The listing builds one solid part. Answer for the finished solid, in the listing's coordinates (mm). A direction names the side the tool comes from. Round coordinates to 2 decimals unless told otherwise and drop trailing zeros. Write each loop counter-clockwise with the first axis right and the second up, starting at its lowest first coordinate (ties: lowest second). Pieces come first, ordered by that corner, then holes. Notation, with made-up numbers: M 50,-19.75 L 96,-19.75 A29 cw 96,16.25 Z; hole C 19,2.5 d4. An arc over 180 degrees is marked long. One line per item, written item: value. Start each with the question number.
(1) Consider probe 1 along Y at (x, z) = (6.25, -1) (3 decimals); probe 2 along Z at (x, y) = (6.25, 2.4) (1 decimal); probe 3 along Z at (x, y) = (11.25, -18.5). Determine where each line is inside the solid, lowest interval first.
(2) Section D-D (x = 10.75) is taken. Determine the outline of the cut face in (y, z) (3 decimals).
(3) For faces 5 (the flat face through (6, -10, -2)), 6 (the flat face through (9, -19.094, -1)), 7 (the flat face through (6, 5, -7)), determine the directions among +Z, -Z, +X, -X, +Y, -Y from which every point of the face is accessible in a straight line to the end or side of a thin tool.
(4) Given P1, Ø3, axis at x = 2, y = -9.5, coming from the -Z side; P2, Ø6, axis at x = 4, z = -9, coming from the -Y side; P3, Ø1, axis at x = 7.5, z = -0.5, coming from the -Y side, each flat-ended and moving along its own axis, determine where each tip first touches the part or whether it passes through.
(5) Section C-C (z = -8) is taken. Determine the outline of the cut face in (x, y).
(6) For a pull along X with two mould halves and no side action, classify faces 1 (the flat face through (12.5, 1, -7)), 2 (the cylindrical face through (6.429, -14.387, -1.014)), 3 (the flat face through (0, 1, -6)), 4 (the flat face through (6, 2, -17.135)) as released by +X, released by -X, zero draft, split by the parting line, or undercut.
(7) Section A-A (y = -15.75) is taken. Determine the outline of the cut face in (x, z) (3 decimals), plus the area to 3 significant figures.
(8) Section B-B (x = 6.25) is taken. Determine the outline of the cut face in (y, z) (1 decimal).
```python
from build123d import *

# Parameters (mm, degrees)
SKETCH1_W                  = 12.5
SKETCH1_H                  = 17.135
TABBASE_DEPTH              = 5
SKETCH2_R                  = 1.375
CHASSISMOUNTINGHOLE_DEPTH  = 5
SKETCH3_W                  = 12.5
SKETCH3_H                  = 26
FRONTTAB_DEPTH             = 5
FRONTMOUNTINGHOLESSKETCH_R = 1.375
FRONTMOUNTINGHOLES_DEPTH   = 5
SKETCH4_W                  = 12.5
SKETCH4_H                  = 21
SKETCH4_R                  = 1.375
CUT_EXTRUDE1_DEPTH         = 3
SKETCH6_W                  = 7.78949329
SKETCH6_H                  = 1.90597399
CUT_EXTRUDE2_DEPTH         = 10
SKETCH7_W                  = 4.71050671
SKETCH7_H                  = 1
CUT_EXTRUDE3_DEPTH         = 10


with BuildPart() as part:
    # Sketch1 → tabBase (new body)
    with BuildSketch(Plane(origin=(0, 0, 0), x_dir=(1, 0, 0), z_dir=(0, 1, 0))):
        with Locations((6.25, 8.5675)):
            Rectangle(SKETCH1_W, SKETCH1_H)
    extrude(amount=TABBASE_DEPTH)

    # Sketch2 → chassisMountingHole (cut)
    with BuildSketch(Plane(origin=(0, 5, 0), x_dir=(1, 0, 0), z_dir=(0, 1, 0))):
        with Locations((6.25, 8.5675)):
            Circle(SKETCH2_R)
    extrude(amount=-CHASSISMOUNTINGHOLE_DEPTH, mode=Mode.SUBTRACT)

    # Sketch3 → frontTab (add)
    with BuildSketch(Plane.XY):
        with Locations((6.25, -8)):
            Rectangle(SKETCH3_W, SKETCH3_H)
    extrude(amount=-FRONTTAB_DEPTH)

    # frontMountingHolesSketch → frontMountingHoles (cut)
    with BuildSketch(Plane(origin=(0, 0, -5), x_dir=(-1, 0, 0), z_dir=(0, 0, -1))):
        with Locations((-6.25, -15.75)):
            Circle(FRONTMOUNTINGHOLESSKETCH_R)
        with Locations((-6.25, -7.75)):
            Circle(FRONTMOUNTINGHOLESSKETCH_R)
    extrude(amount=-FRONTMOUNTINGHOLES_DEPTH, mode=Mode.SUBTRACT)

    # Sketch4 → Cut-Extrude1 (cut)
    with BuildSketch(Plane(origin=(0, 0, -5), x_dir=(-1, 0, 0), z_dir=(0, 0, -1))):
        with Locations((-6.25, -10.5)):
            Rectangle(SKETCH4_W, SKETCH4_H)
        with Locations((-6.25, -15.75)):
            Circle(SKETCH4_R, mode=Mode.SUBTRACT)
        with Locations((-6.25, -7.75)):
            Circle(SKETCH4_R, mode=Mode.SUBTRACT)
    extrude(amount=-CUT_EXTRUDE1_DEPTH, mode=Mode.SUBTRACT)

    # Sketch6 → Cut-Extrude2 (cut)
    with BuildSketch(Plane(origin=(0, 0, -2), x_dir=(-1, 0, 0), z_dir=(0, 0, -1))):
        with Locations((-8.605253355, -20.047013005)):
            Rectangle(SKETCH6_W, SKETCH6_H)
    extrude(amount=-CUT_EXTRUDE2_DEPTH, mode=Mode.SUBTRACT)

    # Sketch7 → Cut-Extrude3 (cut)
    with BuildSketch(Plane(origin=(0, 0, -2), x_dir=(-1, 0, 0), z_dir=(0, 0, -1))):
        with Locations((-2.355253355, -20.5)):
            Rectangle(SKETCH7_W, SKETCH7_H)
    extrude(amount=-CUT_EXTRUDE3_DEPTH, mode=Mode.SUBTRACT)


solid = part.part
```
Recorded:
1. probe 1: y = -19.094 to -17.125, -14.375 to -9.125, -6.375 to 5
1. probe 2: z = -17.1 to -9.9, -7.2 to 0
1. probe 3: z = -2 to 0
2. outline: M -19.094,-2 L 0,-2 L 0,-17.135 L 5,-17.135 L 5,0 L -19.094,0 Z
3. face 5: -Z, +X, -X, -Y
3. face 6: +Z, -Z, +X, -Y
3. face 7: +Z, -Z, +X, -X, +Y
4. P1: stops at z = -2
4. P2: stops at y = 0
4. P3: stops at y = -19.09
5. outline: M 0,0 L 5,0 L 5,5 L 0,5 Z; M 7.5,0 L 12.5,0 L 12.5,5 L 7.5,5 Z
6. face 1: released by +X
6. face 2: undercut
6. face 3: released by -X
6. face 4: zero draft
7. outline: M 0,-2 L 4.875,-2 L 4.875,0 L 0,0 Z; M 7.625,-2 L 12.5,-2 L 12.5,0 L 7.625,0 Z
7. area: 19.5 mm2
8. outline: M -19.1,-2 L -17.1,-2 L -17.1,0 L -19.1,0 Z; M -14.4,-2 L -9.1,-2 L -9.1,0 L -14.4,0 Z; M -6.4,-2 L 0,-2 L 0,-7.2 L 5,-7.2 L 5,0 L -6.4,0 Z; M 0,-17.1 L 5,-17.1 L 5,-9.9 L 0,-9.9 Z
